Verification items for the finished model (mm, model axes). A direction names the side the tool comes from. Round coordinates to 2 decimals unless told otherwise and drop trailing zeros. Write each loop counter-clockwise with the first axis right and the second up, starting at its lowest first coordinate (ties: lowest second). Pieces come first, ordered by that corner, then holes. Notation, with made-up numbers: (-15.5, 21) - (20.5, 21) arc R27 ccw to (20.5, 55) - close; hole circle Ø2 at (26, 21). An arc over 180 degrees is marked (long way). Answer as a JSON object with one key per item and string values.
```python
from build123d import *

# Parameters (mm, degrees)
F0_W     = 25.3
F0_H     = 30
F1_DEPTH = 3
F2_W     = 3
F2_H     = 30
F3_DEPTH = 25
F5_DEPTH = 3
F6_R     = 1
F7_DEPTH = 3


# Not quite as in the source:
# - a feature names something its author has since deleted; it is built from what else it names


with BuildPart() as f1:
    # F0 (on Top) → F1 (new body)
    with BuildSketch(Plane.XY):
        Rectangle(F0_W, F0_H)
    extrude(amount=-F1_DEPTH)

    # F2 (on face) → F3 (join)
    with BuildSketch(Plane.XY):
        with Locations((-11.15, 0)):
            Rectangle(F2_W, F2_H)
    extrude(amount=F3_DEPTH)

    # F4 (on face) → F5 (cut)
    with BuildSketch(Plane(origin=(-12.65, 0, 0), x_dir=(0, -1, 0), z_dir=(-1, 0, 0))):
        with BuildLine():
            ThreePointArc((3, 15), (-2.1213203436, 17.1213203436), (0, 12))
            ThreePointArc((0, 12), (2.1213203436, 12.8786796564), (3, 15))
        make_face()
        with BuildLine():
            Line((-15, 25), (-15, 0))
            Line((-15, 0), (-9.569428978, 17.9027623113))
            ThreePointArc((-9.569428978, 17.9027623113), (-5.9570284911, 23.032049026), (0, 25))
            Line((0, 25), (-15, 25))
        make_face()
        with BuildLine():
            Line((9.569428978, 17.9027623113), (15, 0))
            Line((15, 0), (15, 25))
            Line((15, 25), (0, 25))
            ThreePointArc((0, 25), (5.9570284911, 23.032049026), (9.569428978, 17.9027623113))
        make_face()
    extrude(amount=-F5_DEPTH, mode=Mode.SUBTRACT)

    # F6 (on face) → F7 (cut)
    with BuildSketch(Plane.XY):
        with Locations((7.15, -9.5)):
            Circle(F6_R)
        with Locations((-4.15, 0)):
            Circle(F6_R)
        with Locations((7.15, 9.5)):
            Circle(F6_R)
    extrude(amount=-F7_DEPTH, mode=Mode.SUBTRACT)


solid = f1.part
```
Q1. Section check A-A, the plane x = 7.15. Record the cut outline in (y, z), then the cut area to 3 significant figures.
Geometry check:
{"outline": "(-15, -3) - (-10.5, -3) - (-10.5, 0) - (-15, 0) - close; (-8.5, -3) - (8.5, -3) - (8.5, 0) - (-8.5, 0) - close; (10.5, -3) - (15, -3) - (15, 0) - (10.5, 0) - close", "area": "78.0 mm2"}
Q2. Section check B-B, the plane y = -2.5. Record the cut outline in (x, z), then the cut area to 3 significant figures.
Geometry check:
{"outline": "(-12.65, -3) - (12.65, -3) - (12.65, 0) - (-9.65, 0) - (-9.65, 13.34) - (-12.65, 13.34) - close; (-12.65, 16.66) - (-9.65, 16.66) - (-9.65, 24.68) - (-12.65, 24.68) - close", "area": "140 mm2"}
Q3. Set-up check for faces 1 (the flat face through (0, 0, -3)), 2 (the flat face through (1, 0, 0)): record each of +Z, -Z, +X, -X, +Y, -Y from which the full face is reachable in a straight line by a thin tool's end or side.
Geometry check:
{"face 1": "-Z, +X, -X, +Y, -Y", "face 2": "+Z, +X, +Y, -Y"}
Q4. Release check for a two-part mould opening along Y. For faces 3 (the cylindrical face through (7.02, -8.51, -1.48)), 4 (the flat face through (-9.65, 0, 10)), 5 (the flat face through (0, 15, -2)), 6 (the flat face through (-11.171, -12.247, 9.077)) record: released by +Y, released by -Y, zero draft, split by the parting line, or undercut.
Geometry check:
{"face 3": "undercut", "face 4": "zero draft", "face 5": "released by +Y", "face 6": "released by -Y"}
Q5. Material ranges on line 1 along Y through (x, z) = (7.15, -1.55); line 2 along Y through (x, z) = (-4.15, -0.85); line 3 along X through (y, z) = (-7.25, 16.25), recorded low to high. Write a range as [from, to].
Geometry check:
{"line 1": "y = [-15, -10.5], [-8.5, 8.5], [10.5, 15]", "line 2": "y = [-15, -1], [1, 15]", "line 3": "x = [-12.65, -9.65]"}
Q6. Section check C-C, the plane x = -4.75. Record the cut outline in (y, z).
Geometry check:
{"outline": "(-15, -3) - (-0.8, -3) - (-0.8, 0) - (-15, 0) - close; (0.8, -3) - (15, -3) - (15, 0) - (0.8, 0) - close"}
Q7. Section check D-D, the plane x = 10.5. Record the cut outline in (y, z), then the cut area to 3 significant figures.
Geometry check:
{"outline": "(-15, -3) - (15, -3) - (15, 0) - (-15, 0) - close", "area": "90.0 mm2"}
Q8. Gauge pin test, flat ends, axial feed: P1, Ø7, axis at y = 0, z = 15, coming from the +X side; P2, Ø10, axis at x = -10, z = 13.5, coming from the -Y side; P3, Ø4, axis at y = -8.5, z = 21.5, coming from the -X side; P4, Ø2.5, axis at x = -4.15, y = 0, coming from the +Z side. Record the tip position at first contact, or that the pin passes through.
Geometry check:
{"P1": "stops at x = -9.65", "P2": "stops at y = -12.42", "P3": "stops at x = -12.65", "P4": "stops at z = 0"}
